from build123d import *

# Parameters (mm, degrees)
SKETCH1_W               = 20.2692
SKETCH1_H               = 25.4
BOSS_EXTRUDE1_DEPTH     = 7.6708
SKETCH2_R               = 1.9939
SKETCH2_R_2             = 1.6383
BOSS_EXTRUDE2_DEPTH     = 8.7122
SKETCH3_R               = 1.6383
CUT_EXTRUDE1_DEPTH      = 1
CUT_EXTRUDE1_DEPTH_BACK = 17.383


with BuildPart() as part:
    # Sketch1 → Boss-Extrude1 (new body)
    with BuildSketch(Plane(origin=(0, 0, 0), x_dir=(1, 0, 0), z_dir=(0, 1, 0))):
        with Locations((0.995181162, -4.637001603)):
            Rectangle(SKETCH1_W, SKETCH1_H)
    extrude(amount=BOSS_EXTRUDE1_DEPTH)

    # Sketch2 → Boss-Extrude2 (add)
    with BuildSketch(Plane(origin=(0, 0, 0), x_dir=(-1, 0, 0), z_dir=(0, -1, 0))):
        with Locations((7.01266761, -15.1920941)):
            Circle(SKETCH2_R)
        with Locations((7.01266761, -15.1920941)):
            Circle(SKETCH2_R_2, mode=Mode.SUBTRACT)
        with Locations((-8.925132573, -15.1920941)):
            Circle(SKETCH2_R)
        with Locations((-8.925132573, -15.1920941)):
            Circle(SKETCH2_R_2, mode=Mode.SUBTRACT)
        with Locations((-8.925132573, 5.902511421)):
            Circle(SKETCH2_R)
        with Locations((-8.925132573, 5.902511421)):
            Circle(SKETCH2_R_2, mode=Mode.SUBTRACT)
        with Locations((7.01266761, 5.902511421)):
            Circle(SKETCH2_R)
        with Locations((7.01266761, 5.902511421)):
            Circle(SKETCH2_R_2, mode=Mode.SUBTRACT)
    extrude(amount=BOSS_EXTRUDE2_DEPTH)

    # Sketch3 → Cut-Extrude1 (cut, two sides)
    with BuildSketch(Plane(origin=(0, 7.6708, 0), x_dir=(1, 0, 0), z_dir=(0, 1, 0))) as cut_extrude1_sk:
        with Locations((8.925132573, 5.902511421)):
            Circle(SKETCH3_R)
        with Locations((-7.01266761, 5.902511421)):
            Circle(SKETCH3_R)
        with Locations((8.925132573, -15.1920941)):
            Circle(SKETCH3_R)
        with Locations((-7.01266761, -15.1920941)):
            Circle(SKETCH3_R)
    extrude(amount=CUT_EXTRUDE1_DEPTH, mode=Mode.SUBTRACT)
    extrude(cut_extrude1_sk.sketch, amount=-CUT_EXTRUDE1_DEPTH_BACK, mode=Mode.SUBTRACT)


solid = part.part
Source: CAD feature listing. Evaluate the final solid. Frame: model axes, mm. A direction names the side the tool comes from. Give positions to 0.01 mm unless a question says otherwise; leave off trailing zeros. Write each loop counter-clockwise with the first axis right and the second up, starting at its lowest first coordinate (ties: lowest second). Pieces come first, ordered by that corner, then holes. Notation, with made-up numbers: (43, 4.25) - (94, 4.25) arc R5 cw to (94, 8.25) - close; hole circle Ø4 at (-27.5, 47). An arc over 180 degrees is marked (long way). Write item = value, one per line. Start each with the question number.
Q1. Cut plane D-D, the plane y = 3. Return loops of the section in (x, z).
Q2. Draft query along Z for faces 1 (the flat face through (1, 4, 17.337)), 2 (the flat face through (1, 7.671, 4)), 3 (the cylindrical face through (7.29, -0.41, -5.97)). Return one class per face: +Z half, -Z half, draft (parallel to the pull), parting line (faces both ways), or undercut.
Q3. Cut plane B-B, the plane x = -8. Return loops of the section in (y, z).
Q4. Reachability of faces 4 (the flat face through (-9.139, 4, 5)), 5 (the cylindrical face through (-5.43, -4.3, -4.69)) from +Z, -Z, +X, -X, +Y, -Y: full face, straight path, thin tool, end or side. Return the list, or none.
Q5. Pin query (flat end, axial travel): pin 1 Ø3 at (x, z) = (-7.01, 15.19) entering from +Y; pin 2 Ø1 at (x, z) = (-2.5, 1.5) entering from -Y. Return the tip coordinate at first contact, or that it passes through.
Q6. Cut plane C-C, the plane z = 14.75. Return loops of the section in (x, y).
Q7. Cut plane A-A, the plane y = -4.25. Return loops of the section in (x, z).
Q8. Material intervals for probe 1 along X at (y, z) = (-1.25, 14.75); probe 2 along Z at (x, y) = (7.5, 6.5); probe 3 along Y at (x, z) = (-0.5, 4.5), sorted ascending.
Computed values:
q1.outline = (-9.14, -8.06) - (11.13, -8.06) - (11.13, 17.34) - (-9.14, 17.34) - close; hole circle Ø3.28 at (-7.01, -5.9); hole circle Ø3.28 at (-7.01, 15.19); hole circle Ø3.28 at (8.93, -5.9); hole circle Ø3.28 at (8.93, 15.19)
q2.face_1 = +Z half
q2.face_2 = draft
q2.face_3 = undercut
q3.outline = (-8.71, -7.63) - (0, -7.63) - (0, -8.06) - (7.67, -8.06) - (7.67, -7.21) - (-8.71, -7.21) - close; (-8.71, -4.6) - (7.67, -4.6) - (7.67, 13.88) - (-8.71, 13.88) - (-8.71, 13.46) - (0, 13.46) - (0, -4.17) - (-8.71, -4.17) - close; (-8.71, 16.5) - (7.67, 16.5) - (7.67, 17.34) - (0, 17.34) - (0, 16.92) - (-8.71, 16.92) - close
q4.face_4 = +Z, -Z, -X, +Y, -Y
q4.face_5 = -Y
q5.pin_1 = through
q5.pin_2 = 0
q6.outline = (-9.14, 0) - (-8.96, 0) - (-8.96, -8.71) - (-8.59, -8.71) - (-8.59, 7.67) - (-9.14, 7.67) - close; (-5.44, -8.71) - (-5.07, -8.71) - (-5.07, 0) - (6.98, 0) - (6.98, -8.71) - (7.35, -8.71) - (7.35, 7.67) - (-5.44, 7.67) - close; (10.5, -8.71) - (10.87, -8.71) - (10.87, 0) - (11.13, 0) - (11.13, 7.67) - (10.5, 7.67) - close
q7.outline = circle Ø3.99 at (-7.01, -5.9); circle Ø3.99 at (-7.01, 15.19); circle Ø3.99 at (8.93, -5.9); circle Ø3.99 at (8.93, 15.19); hole circle Ø3.28 at (-7.01, -5.9); hole circle Ø3.28 at (-7.01, 15.19); hole circle Ø3.28 at (8.93, -5.9); hole circle Ø3.28 at (8.93, 15.19)
q8.probe_1 = -8.96 to -8.59, -5.44 to -5.07, 6.98 to 7.35, 10.5 to 10.87
q8.probe_2 = -8.06 to -6.71, -5.09 to 14.38, 16 to 17.34
q8.probe_3 = 0 to 7.67
